from build123d import *

# Parameters (mm, degrees)
EXTRUDE_THIN1_DEPTH = 444.5
FILLET1_R           = 1.27


with BuildPart() as part:
    # Sketch1 → Extrude-Thin1 (new body)
    with BuildSketch(Plane.XY):
        with BuildLine():
            Line((0, 6.35), (0, 0))
            Line((0, 0), (-3.96875, 0))
            ThreePointArc((-3.96875, 0), (-3.690796903, 3.353029057), (-5.164974256, 6.37740716))
            ThreePointArc((-5.164974256, 6.37740716), (-6.806228989, 9.331186698), (-7.070099394, 12.7))
            Line((-7.070099394, 12.7), (-9.525, 12.7))
            Line((-9.525, 12.7), (-9.525, 15.875))
            Line((-9.525, 15.875), (-11.1125, 15.875))
            Line((-11.1125, 15.875), (-11.1125, 44.45))
            Line((-11.1125, 44.45), (-4.7625, 44.45))
            Line((-4.7625, 44.45), (-4.7625, 38.1))
            Line((-4.7625, 38.1), (-6.0325, 38.1))
            Line((-6.0325, 38.1), (-6.0325, 43.18))
            Line((-6.0325, 43.18), (-9.8425, 43.18))
            Line((-9.8425, 43.18), (-9.8425, 17.145))
            Line((-9.8425, 17.145), (-8.255, 17.145))
            Line((-8.255, 17.145), (-8.255, 13.97))
            Line((-8.255, 13.97), (-5.446343041, 13.97))
            ThreePointArc((-5.446343041, 13.97), (-5.765030298, 10.42206557), (-4.211578375, 7.216416274))
            ThreePointArc((-4.211578375, 7.216416274), (-2.654146129, 4.440218432), (-2.366770495, 1.27))
            Line((-2.366770495, 1.27), (-1.27, 1.27))
            Line((-1.27, 1.27), (-1.27, 6.35))
            Line((-1.27, 6.35), (0, 6.35))
        make_face()
    extrude(amount=-EXTRUDE_THIN1_DEPTH)

    # Fillet1
    fillet1_edges = [part.edges().sort_by_distance(p)[0] for p in [
        (-8.255, 17.145, -222.25),
        (-5.446343041, 13.97, -222.25),
        (0, 0, -222.25),
        (-3.96875, 0, -222.25),
        (-9.525, 12.7, -222.25),
        (-11.1125, 15.875, -222.25),
        (-11.1125, 44.45, -222.25),
        (-4.7625, 44.45, -222.25),
    ]]
    fillet(fillet1_edges, radius=FILLET1_R)


solid = part.part
Model file for the job. Use its own axes, mm. Give positions to 0.01 mm unless a question says otherwise; leave off trailing zeros. Order: outer loops, then holes, each group sorted by start corner. A loop starts at its lowest first (then second) coordinate and runs counter-clockwise, first axis right, second up. Notation, with made-up numbers: M 65,-9.75 L 76,-9.75 A22 ccw 76,-3.75 Z; hole C 22.5,27.5 d6. An arc over 180 degrees is marked long. Put each result on its own line as item: value. Start each with the question number.
(1) Pull direction Y, two halves, no side cores. Call faces 1 (the face through (-10, 22, -444.5)), 2 (the face through (-9.842, 30, -219)): released by +Y, released by -Y, zero draft, split by the parting line, or undercut.
(2) Band-saw the part on B-B on y = 30.5. Give the cut face in (x, z), then the cut area to 3 significant figures.
(3) Pin check, flat tips, straight feed: pin 1 Ø0.5 at (x, z) = (-2, -204.5) entering from +Y; pin 2 Ø21 at (y, z) = (24.5, -248) entering from +X (3 decimals); pin 3 Ø5.5 at (y, z) = (40, -305.5) entering from +X; pin 4 Ø5 at (x, y) = (-6, 34.5) entering from -Z. Stop position of each tip, or through.
(4) Drill centre lines: L1, parallel to X at y = 41, z = -162; L2, parallel to Y at x = -8, z = -61; L3, parallel to X at y = 5.5, z = -38.5. Where is each one in solid material? Low to high. Write a range as [from, to].
Results below:
1. face 1: zero draft
1. face 2: undercut
2. outline: M -11.11,-444.5 L -9.84,-444.5 L -9.84,0 L -11.11,0 Z
2. area: 565 mm2
3. pin 1: stops at y = 1.27
3. pin 2: stops at x = -8.255
3. pin 3: stops at x = -4.76
3. pin 4: passes through
4. L1: x = [-11.11, -9.84], [-6.03, -4.76]
4. L2: y = [12.7, 13.97], [43.18, 44.45]
4. L3: x = [-4.52, -3.07], [-1.27, 0]
